Check sheet for the modelled part. Datum: model origin and axes. Units: mm. Give positions to 0.01 mm unless a question says otherwise; leave off trailing zeros. Write each loop counter-clockwise with the first axis right and the second up, starting at its lowest first coordinate (ties: lowest second). Pieces come first, ordered by that corner, then holes. Notation, with made-up numbers: (-39, 11) -> (-27, 11) arc R28 cw to (-27, 32) -> close; hole circle Ø11 at (68.25, 9.25). An arc over 180 degrees is marked (long way). Answer as a JSON object with one key per item and string values.
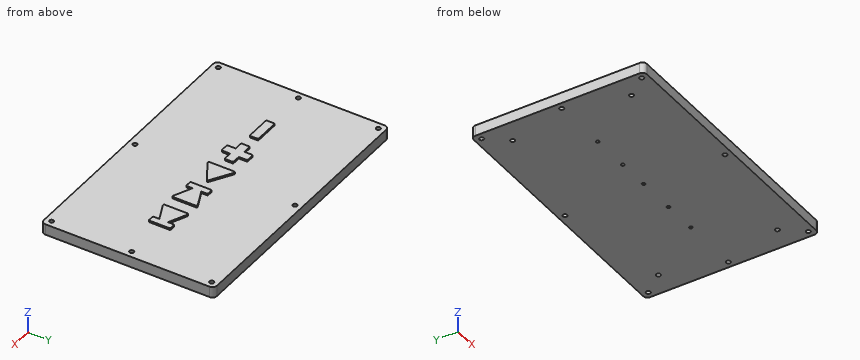
from build123d import *

# Parameters (mm, degrees)
BOSS_EXTRUDE1_DEPTH = 5
BOSS_EXTRUDE2_DEPTH = 0.8
SKETCH22_R          = 0.75
CUT_EXTRUDE1_DEPTH  = 1
SKETCH18_R          = 1
CUT_EXTRUDE2_DEPTH  = 35
SKETCH15_R          = 1
CUT_EXTRUDE3_DEPTH  = 3


with BuildPart() as part:
    # Sketch1 → Boss-Extrude1 (new body)
    with BuildSketch(Plane.XY):
        with BuildLine():
            Line((-61, 40), (61, 40))
            ThreePointArc((61, 40), (62.414213562, 39.414213562), (63, 38))
            Line((63, 38), (63, -38))
            ThreePointArc((63, -38), (62.414213562, -39.414213562), (61, -40))
            Line((61, -40), (-61, -40))
            ThreePointArc((-61, -40), (-62.414213562, -39.414213562), (-63, -38))
            Line((-63, -38), (-63, 38))
            ThreePointArc((-63, 38), (-62.414213562, 39.414213562), (-61, 40))
        make_face()
    extrude(amount=BOSS_EXTRUDE1_DEPTH)

    # Sketch19 → Boss-Extrude2 (add)
    with BuildSketch(Plane.XY.offset(5)):
        with BuildLine():
            Line((-5, 5.7), (-5, -5.7))
            ThreePointArc((-5, -5.7), (-4.746349407, -6.135099953), (-4.242752122, -6.128746463))
            Line((-4.242752122, -6.128746463), (5.257247878, -0.428746463))
            ThreePointArc((5.257247878, -0.428746463), (5.5, 0), (5.257247878, 0.428746463))
            Line((5.257247878, 0.428746463), (-4.242752122, 6.128746463))
            ThreePointArc((-4.242752122, 6.128746463), (-4.746349407, 6.135099953), (-5, 5.7))
        make_face()
        with BuildLine():
            Line((-10, -1.5), (-10, 1.5))
            ThreePointArc((-10, 1.5), (-10.146446609, 1.853553391), (-10.5, 2))
            Line((-10.5, 2), (-14, 2))
            Line((-14, 2), (-14, 5.5))
            ThreePointArc((-14, 5.5), (-14.146446609, 5.853553391), (-14.5, 6))
            Line((-14.5, 6), (-17.5, 6))
            ThreePointArc((-17.5, 6), (-17.853553391, 5.853553391), (-18, 5.5))
            Line((-18, 5.5), (-18, 2))
            Line((-18, 2), (-21.5, 2))
            ThreePointArc((-21.5, 2), (-21.853553391, 1.853553391), (-22, 1.5))
            Line((-22, 1.5), (-22, -1.5))
            ThreePointArc((-22, -1.5), (-21.853553391, -1.853553391), (-21.5, -2))
            Line((-21.5, -2), (-18, -2))
            Line((-18, -2), (-18, -5.5))
            ThreePointArc((-18, -5.5), (-17.853553391, -5.853553391), (-17.5, -6))
            Line((-17.5, -6), (-14.5, -6))
            ThreePointArc((-14.5, -6), (-14.146446609, -5.853553391), (-14, -5.5))
            Line((-14, -5.5), (-14, -2))
            Line((-14, -2), (-10.5, -2))
            ThreePointArc((-10.5, -2), (-10.146446609, -1.853553391), (-10, -1.5))
        make_face()
        with BuildLine():
            Line((-28, 1.5), (-28, -1.5))
            ThreePointArc((-28, -1.5), (-28.146446609, -1.853553391), (-28.5, -2))
            Line((-28.5, -2), (-39.5, -2))
            ThreePointArc((-39.5, -2), (-39.853553391, -1.853553391), (-40, -1.5))
            Line((-40, -1.5), (-40, 1.5))
            ThreePointArc((-40, 1.5), (-39.853553391, 1.853553391), (-39.5, 2))
            Line((-39.5, 2), (-28.5, 2))
            ThreePointArc((-28.5, 2), (-28.146446609, 1.853553391), (-28, 1.5))
        make_face()
        with BuildLine():
            Line((10, 4.5), (10, -4.5))
            ThreePointArc((10, -4.5), (10.146446609, -4.853553391), (10.5, -5))
            Line((10.5, -5), (12.5, -5))
            ThreePointArc((12.5, -5), (12.853553391, -4.853553391), (13, -4.5))
            Line((13, -4.5), (13, -2))
            Line((13, -2), (21.296930767, -5.687524785))
            ThreePointArc((21.296930767, -5.687524785), (21.77245677, -5.64986513), (22, -5.230619011))
            Line((22, -5.230619011), (22, 5.230619011))
            ThreePointArc((22, 5.230619011), (21.77245677, 5.64986513), (21.296930767, 5.687524785))
            Line((21.296930767, 5.687524785), (13, 2))
            Line((13, 2), (13, 4.5))
            ThreePointArc((13, 4.5), (12.853553391, 4.853553391), (12.5, 5))
            Line((12.5, 5), (10.5, 5))
            ThreePointArc((10.5, 5), (10.146446609, 4.853553391), (10, 4.5))
        make_face()
        with BuildLine():
            Line((28, 5.230619011), (28, -5.230619011))
            ThreePointArc((28, -5.230619011), (28.22754323, -5.64986513), (28.703069233, -5.687524785))
            Line((28.703069233, -5.687524785), (37, -2))
            Line((37, -2), (37, -4.5))
            ThreePointArc((37, -4.5), (37.146446609, -4.853553391), (37.5, -5))
            Line((37.5, -5), (39.5, -5))
            ThreePointArc((39.5, -5), (39.853553391, -4.853553391), (40, -4.5))
            Line((40, -4.5), (40, 4.5))
            ThreePointArc((40, 4.5), (39.853553391, 4.853553391), (39.5, 5))
            Line((39.5, 5), (37.5, 5))
            ThreePointArc((37.5, 5), (37.146446609, 4.853553391), (37, 4.5))
            Line((37, 4.5), (37, 2))
            Line((37, 2), (28.703069233, 5.687524785))
            ThreePointArc((28.703069233, 5.687524785), (28.22754323, 5.64986513), (28, 5.230619011))
        make_face()
    extrude(amount=BOSS_EXTRUDE2_DEPTH)

    # Sketch22 → Cut-Extrude1 (cut)
    with BuildSketch(Plane.XY):
        with Locations((-34, 0)):
            Circle(SKETCH22_R)
        with Locations((-16, 0)):
            Circle(SKETCH22_R)
        with Locations((-1, 0)):
            Circle(SKETCH22_R)
        with Locations((17, 0)):
            Circle(SKETCH22_R)
        with Locations((33, 0)):
            Circle(SKETCH22_R)
    extrude(amount=CUT_EXTRUDE1_DEPTH, mode=Mode.SUBTRACT)

    # Sketch18 → Cut-Extrude2 (cut)
    with BuildSketch(Plane.XY):
        with Locations((60, 37)):
            Circle(SKETCH18_R)
        with Locations((60, -37)):
            Circle(SKETCH18_R)
        with Locations((-60, -37)):
            Circle(SKETCH18_R)
        with Locations((-60, 37)):
            Circle(SKETCH18_R)
        with Locations((0, 37)):
            Circle(SKETCH18_R)
        with Locations((0, -37)):
            Circle(SKETCH18_R)
        with Locations((-60, 0)):
            Circle(SKETCH18_R)
        with Locations((60, 0)):
            Circle(SKETCH18_R)
    extrude(amount=CUT_EXTRUDE2_DEPTH, mode=Mode.SUBTRACT)

    # Sketch15 → Cut-Extrude3 (cut)
    with BuildSketch(Plane.XY):
        with Locations((-52.5, -27.5)):
            Circle(SKETCH15_R)
        with Locations((-52.5, 27.5)):
            Circle(SKETCH15_R)
        with Locations((52.5, -27.5)):
            Circle(SKETCH15_R)
        with Locations((52.5, 27.5)):
            Circle(SKETCH15_R)
    extrude(amount=CUT_EXTRUDE3_DEPTH, mode=Mode.SUBTRACT)


solid = part.part
1. Sectioned sample at A-A, the plane x = 47.5. Enter the section's corners in (y, z).
Determined:
{"outline": "(-40, 0) -> (40, 0) -> (40, 5) -> (-40, 5) -> close"}
2. Go/stop test with flat-tipped pins: P1, Ø0.9, axis at x = -15.5, z = 5.5, coming from the -Y side; P2, Ø0.9, axis at y = 0, z = 5.5, coming from the +X side; P3, Ø0.6, axis at y = -4, z = 5.5, coming from the -X side. Record where each tip stops, or that it passes through.
Determined:
{"P1": "y = -6", "P2": "x = 40", "P3": "x = -18"}
3. Sectioned sample at B-B, the plane y = 20.5. Enter the section's corners in (x, z), plus the area to 3 significant figures.
Determined:
{"outline": "(-63, 0) -> (63, 0) -> (63, 5) -> (-63, 5) -> close", "area": "630 mm^2"}
4. Scan lines: L1, parallel to Y at x = 60, z = 1.95; L2, parallel to X at y = 0, z = 3; L3, parallel to X at y = 37, z = 2.35. Record each from-to range of solid material in increasing order. Write a range as [from, to].
Determined:
{"L1": "[-40, -38], [-36, -1], [1, 36], [38, 40]", "L2": "[-63, -61], [-59, 59], [61, 63]", "L3": "[-63, -61], [-59, -1], [1, 59], [61, 63]"}
